from build123d import *

# Parameters (mm, degrees)
SKETCH_W  = 230
SKETCH_H  = 220
SKETCH_R  = 2.5
PAD_DEPTH = 2
FILLET_R  = 5


with BuildPart() as part:
    # Sketch → Pad (new body)
    with BuildSketch(Plane.YZ):
        with Locations((10, -10)):
            Rectangle(SKETCH_W, SKETCH_H)
        with Locations((-100, 95)):
            Circle(SKETCH_R, mode=Mode.SUBTRACT)
        with Locations((120, 95)):
            Circle(SKETCH_R, mode=Mode.SUBTRACT)
        with Locations((-100, -115)):
            Circle(SKETCH_R, mode=Mode.SUBTRACT)
        with Locations((120, -115)):
            Circle(SKETCH_R, mode=Mode.SUBTRACT)
    extrude(amount=PAD_DEPTH)

    # Fillet
    fillet_edges = [part.edges().sort_by_distance(p)[0] for p in [
        (1, 125, -120),
        (1, -105, -120),
        (1, -105, 100),
        (1, 125, 100),
    ]]
    fillet(fillet_edges, radius=FILLET_R)


solid = part.part
Model file for the job. Use its own axes, mm. Round coordinates to 2 decimals unless told otherwise and drop trailing zeros. Answer as CSV lines item,"result". Start each with the question number.
1) Pin check, flat tip, straight feed: P1, Ø12, axis at y = -61, z = 38.5, coming from the -X side. Stop position of the tip, or through.
2) Probe line 1 along Z through (x, y) = (1, 120). List the from-to ranges inside material, lowest first.
3) Mould opens along Z. For faces 1 (the face through (1, -104, 98)), 2 (the face through (0.986, 122.385, 95.751)), 3 (the face through (0, 8, -8)) say: +Z half, -Z half, draft (parallel to the pull), parting line (faces both ways), or undercut.
Filled in:
1,P1,"stops at x = 0"
2,line 1,"z = -120 to -117.5, -112.5 to 92.5, 97.5 to 100"
3,face 1,"+Z half"
3,face 2,"undercut"
3,face 3,"draft"
